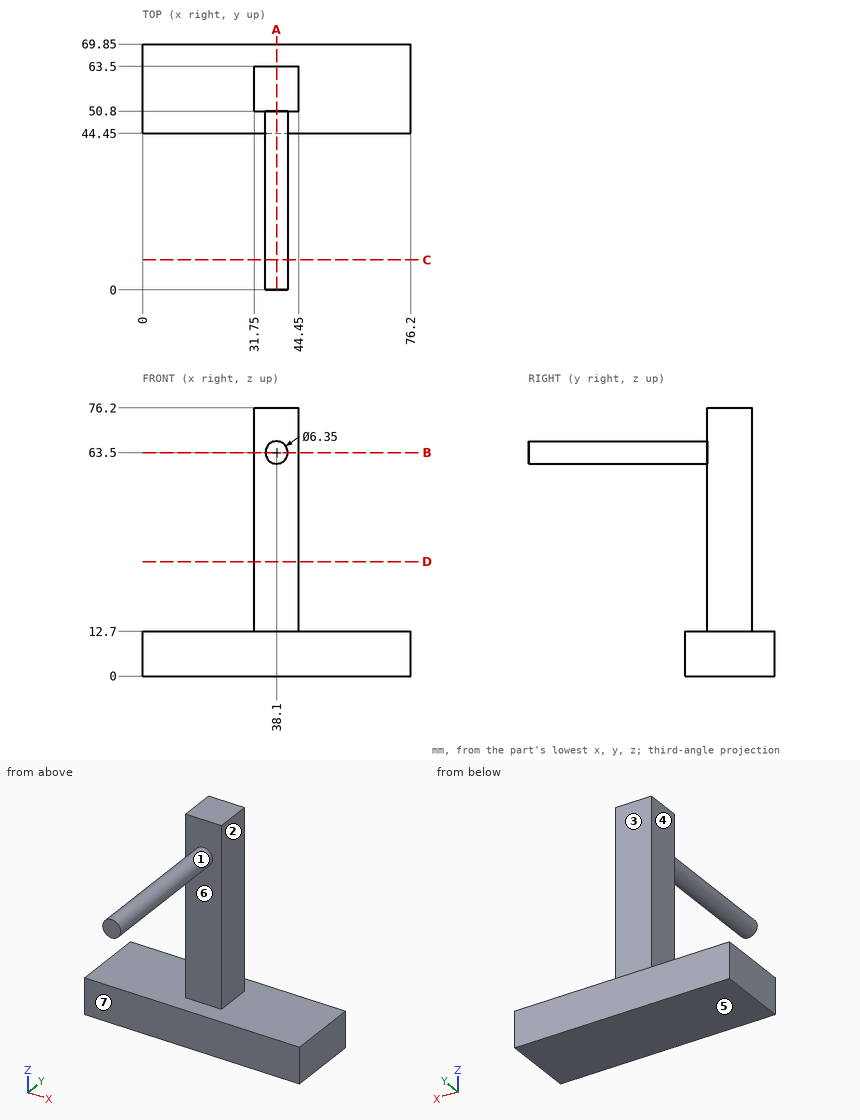
For this review, use the dimensioned drawing (mm, ordinates from the lowest corner) and the shaded views. A direction names the side the tool comes from. Coordinates: 2 decimals unless noted, no trailing zeros. Write each loop counter-clockwise with the first axis right and the second up, starting at its lowest first coordinate (ties: lowest second). Pieces come first, ordered by that corner, then holes. Notation, with made-up numbers: (60.5, 3) -> (78.5, 3) arc R15 ccw to (78.5, 29) -> close; hole circle Ø8 at (-40, -22). An arc over 180 degrees is marked (long way). Put each result on its own line as item: value.
Q1. Clearance check with flat-ended pins moving along their axes: pin 1 Ø10 at (x, z) = (36, 43) entering from +Y; pin 2 Ø6.5 at (y, z) = (54, 54) entering from +X; pin 3 Ø10 at (x, z) = (49, 35) entering from -Y. State where each tip first meets the part, or that it passes through.
From the geometry:
pin 1: stops at y = 63.5
pin 2: stops at x = 44.45
pin 3: stops at y = 50.8
Q2. Take a section at A-A, the plane x = 38.1. State the section outline as (y, z) points (3 decimals).
From the geometry:
outline: (0, 60.325) -> (50.8, 60.325) -> (50.8, 12.7) -> (44.45, 12.7) -> (44.45, 0) -> (69.85, 0) -> (69.85, 12.7) -> (63.5, 12.7) -> (63.5, 76.2) -> (50.8, 76.2) -> (50.8, 66.675) -> (0, 66.675) -> close
Q3. Wall thickness on L1, parallel to X at y = 60, z = 65; L2, parallel to Y at x = 63.5, z = 11; L3, parallel to Y at x = 43.5, z = 34.5: over which ranges is each line inside the solid? List them lowest first.
From the geometry:
L1: x = 31.75 to 44.45
L2: y = 44.45 to 69.85
L3: y = 50.8 to 63.5
Q4. Take a section at D-D, the plane z = 32.5. State the section outline as (x, y) points.
From the geometry:
outline: (31.75, 50.8) -> (44.45, 50.8) -> (44.45, 63.5) -> (31.75, 63.5) -> close
Q5. The part is to be moulded in two halves that separate along Z. For the marked faces 5, 6 and 7, say which applies: +Z half, -Z half, draft (parallel to the pull), parting line (faces both ways), or undercut.
From the geometry:
face 5: -Z half
face 6: undercut
face 7: draft
Q6. Take a section at C-C, the plane y = 8.5. State the section outline as (x, z) points (3 decimals), then the cut area to 3 significant figures.
From the geometry:
outline: circle Ø6.35 at (38.1, 63.5)
area: 31.7 mm2
Q7. Tool access review of the marked faces 1, 2, 3 and 4: name each direction out of +Z, -Z, +X, -X, +Y, -Y from which nothing blocks a thin tool from reaching the whole face with its end or side.
From the geometry:
face 1: -Y
face 2: +Z, +X, +Y, -Y
face 3: +Z, +X, -X, +Y
face 4: +Z, -X, +Y, -Y
Q8. Take a section at B-B, the plane z = 63.5. State the section outline as (x, y) points (3 decimals), then the cut area to 3 significant figures.
From the geometry:
outline: (31.75, 50.8) -> (34.925, 50.8) -> (34.925, 0) -> (41.275, 0) -> (41.275, 50.8) -> (44.45, 50.8) -> (44.45, 63.5) -> (31.75, 63.5) -> close
area: 484 mm2
